Part model, mm, in its own coordinate system. Round coordinates to 2 decimals unless told otherwise and drop trailing zeros. Loops run counter-clockwise (first coordinate to the right, second up) from the corner with the lowest first, then second, coordinate; pieces in that order, holes last. Notation, with made-up numbers: M -10,-38.5 L 8,-38.5 A11 ccw 8,-21.5 Z; hole C -33,30 d8. An arc over 180 degrees is marked long. Answer as CSV lines item,"result". Start each with the question number.
Item 1: Band-saw the part on A-A (y = -8). Give the cut face in (x, z), and give its area (3 significant figures).
Item 2: Drop flat-ended pins along their axis: pin 1 Ø1.4 at (x, z) = (6, -1) entering from +Y; pin 2 Ø5 at (x, z) = (3, -3.5) entering from -Y; pin 3 Ø5 at (x, z) = (6, -1) entering from -Y. Give the stop position or say it passes through.
Item 3: Wall check: line 1 (Y direction, x = -2.5, z = -1.5); line 2 (Y direction, x = 1.5, z = 6.5); line 3 (X direction, y = 3.25, z = -2.5). Give the ranges that are in metal, low to high.
```python
from build123d import *

# Parameters (mm, degrees)
SKETCH_2_R          = 4.4
CUT_EXTRUDE_1_DEPTH = 15
SKETCH_3_W          = 10.421641006
SKETCH_3_H          = 1
CUT_EXTRUDE_2_DEPTH = 15
FILLET_1_R          = 1


with BuildPart() as part:
    # 스케치1 → 회전2 (revolve)
    with BuildSketch(Plane.XY):
        with BuildLine():
            Line((0, 10), (0, -10))
            ThreePointArc((0, -10), (-10, 0), (0, 10))
        make_face()
    revolve(axis=Axis((0, 11.789684906, 0), (0, -1, 0)))

    # 스케치2 → 컷-돌출1 (cut, symmetric)
    with BuildSketch(Plane.XY):
        with Locations(Location((0, 0, 0), (0, 0, 180))):
            Circle(SKETCH_2_R)
    extrude(amount=CUT_EXTRUDE_1_DEPTH, both=True, mode=Mode.SUBTRACT)

    # 스케치3 → 컷-돌출2 (cut, symmetric)
    with BuildSketch(Plane.XY):
        with Locations((6.647452601, 0)):
            Rectangle(SKETCH_3_W, SKETCH_3_H)
    extrude(amount=CUT_EXTRUDE_2_DEPTH, both=True, mode=Mode.SUBTRACT)

    # 필렛1
    fillet_1_edges = [part.edges().sort_by_distance(p)[0] for p in [
        (-0.250405834, -4.392868837, 8.979977728),
        (9.987492178, 0.5, 0),
        (9.987492178, -0.5, 0),
        (-0.250405834, -4.392868837, -8.979977728),
    ]]
    fillet(fillet_1_edges, radius=FILLET_1_R)


solid = part.part
```
Answer block:
1,outline,"C 0,0 d12"
1,area,"113 mm^2"
2,pin 1,"stops at y = 8.43"
2,pin 2,"stops at y = -9.77"
2,pin 3,"stops at y = -9.34"
3,line 1,"y = -9.57 to -3.62, 3.62 to 9.57"
3,line 2,"y = -7.45 to -4.14, 4.14 to 7.45"
3,line 3,"x = -9.12 to -2.97, 2.97 to 9.12"
